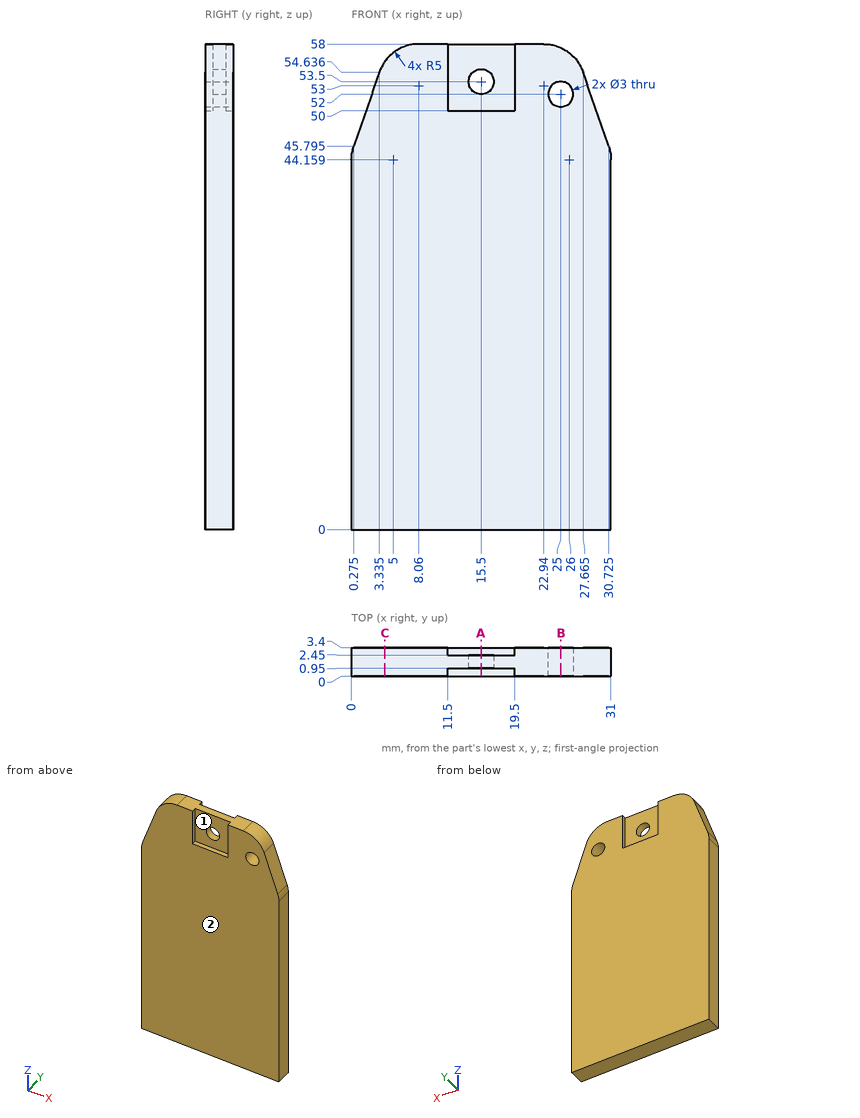
Answer from the drawing. Dimensions are ordinates in mm from the lowest x, y and z of the part. Round coordinates to 2 decimals unless told otherwise and drop trailing zeros. Write each loop counter-clockwise with the first axis right and the second up, starting at its lowest first coordinate (ties: lowest second). Pieces come first, ordered by that corner, then holes. Notation, with made-up numbers: M 9,56.25 L 13,56.25 A17 ccw 13,61.25 Z; hole C -1,57.5 d2. An arc over 180 degrees is marked long. Write each question's results on one line, items separated by ' | '. Start each with the question number.
Item 1: Straight lines are drawn through the part: probe 1 along Z at (x, y) = (15.5, 1.85); probe 2 along Z at (x, y) = (25, 0.6) (1 decimal); probe 3 along Z at (x, y) = (15, 0.45). For each, find the intervals that lie inside material, in ascending order.
Item 2: The mould has two halves that part along X. Classify the marked faces 1 and 2: +X half, -X half, draft (parallel to the pull), parting line (faces both ways), or undercut.
Item 3: Given pin 1 Ø1 at (y, z) = (0.5, 51) entering from +X; pin 2 Ø3.5 at (x, z) = (15.5, 53.5) entering from -Y; pin 3 Ø2.5 at (x, z) = (17.5, 52.5) entering from +Y; pin 4 Ø4 at (x, z) = (25, 52) entering from -Y, each flat-ended and moving along its own axis, determine where each tip first touches the part or whether it passes through.
Item 4: Find section C-C on x = 4. Write down the section's boundary in (y, z), and give its area (3 significant figures).
Item 5: Find section B-B on x = 25. Write down the section's boundary in (y, z) (1 decimal).
Item 6: Find section A-A on x = 15.5. Write down the section's boundary in (y, z).
Answer block:
1) probe 1: z = 0 to 52, 55 to 58 | probe 2: z = 0 to 50.5, 53.5 to 57.6 | probe 3: z = 0 to 50
2) face 1: undercut | face 2: draft
3) pin 1: stops at x = 29.1 | pin 2: stops at y = 0.95 | pin 3: stops at y = 2.45 | pin 4: stops at y = 0
4) outline: M 0,0 L 3.4,0 L 3.4,55.92 L 0,55.92 Z | area: 190 mm²
5) outline: M 0,0 L 3.4,0 L 3.4,50.5 L 0,50.5 Z; M 0,53.5 L 3.4,53.5 L 3.4,57.6 L 0,57.6 Z
6) outline: M 0,0 L 3.4,0 L 3.4,50 L 2.45,50 L 2.45,52 L 0.95,52 L 0.95,50 L 0,50 Z; M 0.95,55 L 2.45,55 L 2.45,58 L 0.95,58 Z
